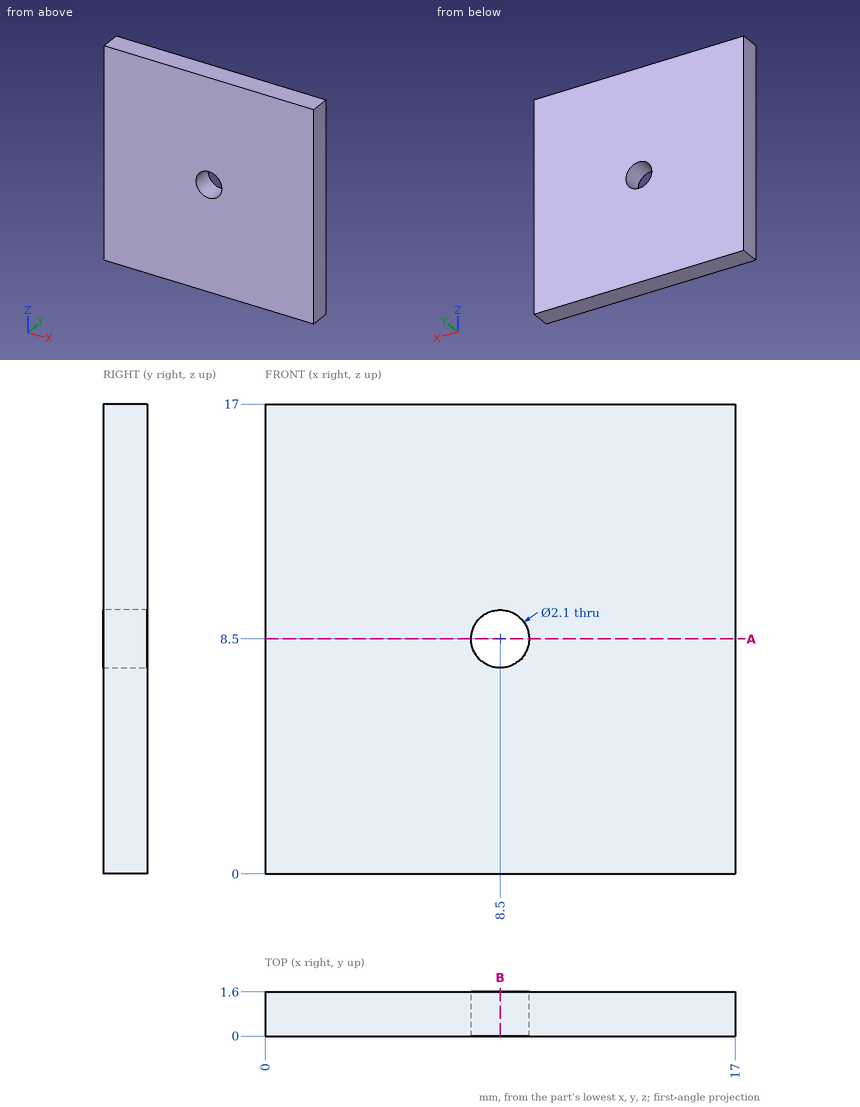
Can you work these out from the drawing? Everything is in mm from the part's minimum corner. Round coordinates to 2 decimals unless told otherwise and drop trailing zeros. Order: outer loops, then holes, each group sorted by start corner. A loop starts at its lowest first (then second) coordinate and runs counter-clockwise, first axis right, second up. Notation, with made-up numbers: M 83,63 L 126,63 A32 ccw 126,95 Z; hole C -22,57.25 d1. An arc over 180 degrees is marked long. Answer as CSV lines item,"result".
Item 1: Please list where these lines run through material, in increasing order: L1, parallel to X at y = 0.5, z = 8.5; L2, parallel to X at y = 0.15, z = 9. Write a range as [from, to].
From the geometry:
L1,"[0, 7.45], [9.55, 17]"
L2,"[0, 7.58], [9.42, 17]"
Item 2: Imagine slicing it at B-B on x = 8.5. List the corners of the cut face in (y, z) for me, and give its area (3 significant figures).
From the geometry:
outline,"M 0,0 L 1.6,0 L 1.6,7.45 L 0,7.45 Z; M 0,9.55 L 1.6,9.55 L 1.6,17 L 0,17 Z"
area,"23.8 mm2"
Item 3: Imagine slicing it at A-A on z = 8.5. List the corners of the cut face in (x, y) for me.
From the geometry:
outline,"M 0,0 L 7.45,0 L 7.45,1.6 L 0,1.6 Z; M 9.55,0 L 17,0 L 17,1.6 L 9.55,1.6 Z"
